Read the model definition and answer for the solid it produces. Units are mm, in the model's axes. A direction names the side the tool comes from. Coordinates: 2 decimals unless noted, no trailing zeros. Write each loop counter-clockwise with the first axis right and the second up, starting at its lowest first coordinate (ties: lowest second). Pieces come first, ordered by that corner, then holes. Notation, with made-up numbers: (55.5, 0) -> (82.5, 0) arc R14 ccw to (82.5, 15) -> close; hole circle Ø1 at (-26, 50). An arc over 180 degrees is marked (long way). Answer as a JSON object with one key per item and string values. Group by question number.
(1) Find section B-B (z = -23). Give the vertices of the cut face in (x, y), then the cut area to 3 significant figures.
(2) Flat-ended cylindrical pins translate along their axes: P1, Ø10, axis at x = -43, z = -7.5, coming from the +Y side; P2, Ø7.5, axis at x = 67.5, y = 144, coming from the +Z side; P3, Ø3, axis at x = -57, y = 120.5, coming from the +Z side. Find the tip coordinate at first contact, or state that the pin passes through.
(3) Which of the six approach directions +Z, -Z, +X, -X, +Y, -Y give full straight-line access (tool end or side, diameter ignored) to faces 5 (the face through (-1, 100, -47.114)), 6 (the face through (-76.2, 100, -2))?
(4) Find section C-C (y = 55). Give the vertices of the cut face in (x, z), then the cut area to 3 significant figures.
(5) Find section D-D (x = -72). Give the vertices of the cut face in (y, z).
(6) For a pull along X with two mould halves and no side action, classify faces 1 (the face through (101.6, 100, -11)), 2 (the face through (-101.6, 100, -10)), 3 (the face through (-63, 100, -31.874)), 4 (the face through (-89, 89, 47.114)) as +X half, -X half, draft (parallel to the pull), parting line (faces both ways), or undercut.
(7) Straight lines are drawn through the part: L1, parallel to X at y = 120, z = 38; L2, parallel to X at y = 124.5, z = 4; L3, parallel to X at y = 110, z = -14.5. For each, find the intervals that lie inside material, in ascending order.
(8) Find section A-A (z = 25.5). Give the vertices of the cut face in (x, y).
from build123d import *

# Parameters (mm, degrees)
F1_DEPTH  = 203.2
F3_W      = 243.94399
F3_H      = 236.642776
F4_DEPTH  = 50.8
F5_W      = 239.845752
F5_H      = 209.126156
F6_DEPTH  = 2.54
F8_W      = 249.582366
F8_H      = 241.68387
F9_DEPTH  = 76.2
F10_W     = 220.484912
F10_H     = 208.068371
F11_DEPTH = 2.54


with BuildPart() as f1:
    # F0 (on Front) → F1 (new body)
    with BuildSketch(Plane.XZ):
        with BuildLine():
            Line((-101.6, -47.114426), (101.6, -47.114426))
            Line((101.6, -47.114426), (101.6, 47.114426))
            Line((101.6, 47.114426), (76.2, 47.114426))
            Line((76.2, 47.114426), (76.2, -31.75))
            Line((76.2, -31.75), (50.8, -31.75))
            ThreePointArc((50.8, -31.75), (-0.064147, 20.566733), (-50.8, -31.874426))
            Line((-50.8, -31.874426), (-76.2, -31.874426))
            Line((-76.2, -31.874426), (-76.2, 47.114426))
            Line((-76.2, 47.114426), (-101.6, 47.114426))
            Line((-101.6, 47.114426), (-101.6, -31.874426))
            Line((-101.6, -31.874426), (-101.6, -47.114426))
        make_face()
    extrude(amount=-F1_DEPTH)

    # F3 (on face) → F4 (cut)
    with BuildSketch(Plane(origin=(0, 14.976081, -10.486365), x_dir=(1, 0, 0), z_dir=(0, -0.819152, 0.573576))):
        with Locations((0, 12.914947)):
            Rectangle(F3_W, F3_H)
    extrude(amount=F4_DEPTH, mode=Mode.SUBTRACT)

    # F5 (on face) → F6 (cut)
    with BuildSketch(Plane(origin=(0, 14.976081, -10.486365), x_dir=(1, 0, 0), z_dir=(0, -0.819152, 0.573576))):
        with Locations((0, 12.164494)):
            Rectangle(F5_W, F5_H)
    extrude(amount=-F6_DEPTH, mode=Mode.SUBTRACT)

    # F8 (on face) → F9 (cut)
    with BuildSketch(Plane(origin=(0, 85.725, 85.725), x_dir=(1, 0, 0), z_dir=(0, -0.707107, -0.707107))):
        with Locations((0, -104.242772)):
            Rectangle(F8_W, F8_H)
    extrude(amount=-F9_DEPTH, mode=Mode.SUBTRACT)

    # F10 (on face) → F11 (cut)
    with BuildSketch(Plane(origin=(0, 85.725, 85.725), x_dir=(1, 0, 0), z_dir=(0, -0.707107, -0.707107))):
        with Locations((0, -103.083611)):
            Rectangle(F10_W, F10_H)
    extrude(amount=F11_DEPTH, mode=Mode.SUBTRACT)


solid = f1.part
Results below:
{
 "1": {"outline": "(-101.6, 9.31) -> (-76.2, 9.31) -> (-76.2, 190.86) -> (-101.6, 190.86) -> close; (-50.3, 9.31) -> (50.3, 9.31) -> (50.3, 190.86) -> (-50.3, 190.86) -> close; (76.2, 9.31) -> (101.6, 9.31) -> (101.6, 190.86) -> (76.2, 190.86) -> close", "area": "27,500 mm2"},
 "2": {"P1": "stops at y = 180.36", "P2": "stops at z = -31.75", "P3": "stops at z = -31.87"},
 "3": {"face 5": "-Z, +X, -X, +Y, -Y", "face 6": "+Z, +Y, -Y"},
 "4": {"outline": "(-101.6, -47.11) -> (101.6, -47.11) -> (101.6, 42.25) -> (76.2, 42.25) -> (76.2, -31.75) -> (50.8, -31.75) arc R50.82 ccw (long way) to (-50.8, -31.87) -> (-76.2, -31.87) -> (-76.2, 42.25) -> (-101.6, 42.25) -> close", "area": "11,100 mm2"},
 "5": {"outline": "(0, -47.11) -> (203.2, -47.11) -> (203.2, -35.34) -> (199.73, -31.87) -> (3.1, -31.87) -> (0, -36.3) -> close"},
 "6": {"face 1": "+X half", "face 2": "-X half", "face 3": "undercut", "face 4": "draft"},
 "7": {"L1": "x = -101.6 to -76.2, 76.2 to 101.6", "L2": "x = -101.6 to -76.2, -37.55 to 37.54, 76.2 to 101.6", "L3": "x = -101.6 to -76.2, -48.32 to 48.32, 76.2 to 101.6"},
 "8": {"outline": "(-101.6, 43.27) -> (-76.2, 43.27) -> (-76.2, 142.36) -> (-101.6, 142.36) -> close; (76.2, 43.27) -> (101.6, 43.27) -> (101.6, 142.36) -> (76.2, 142.36) -> close"}
}
